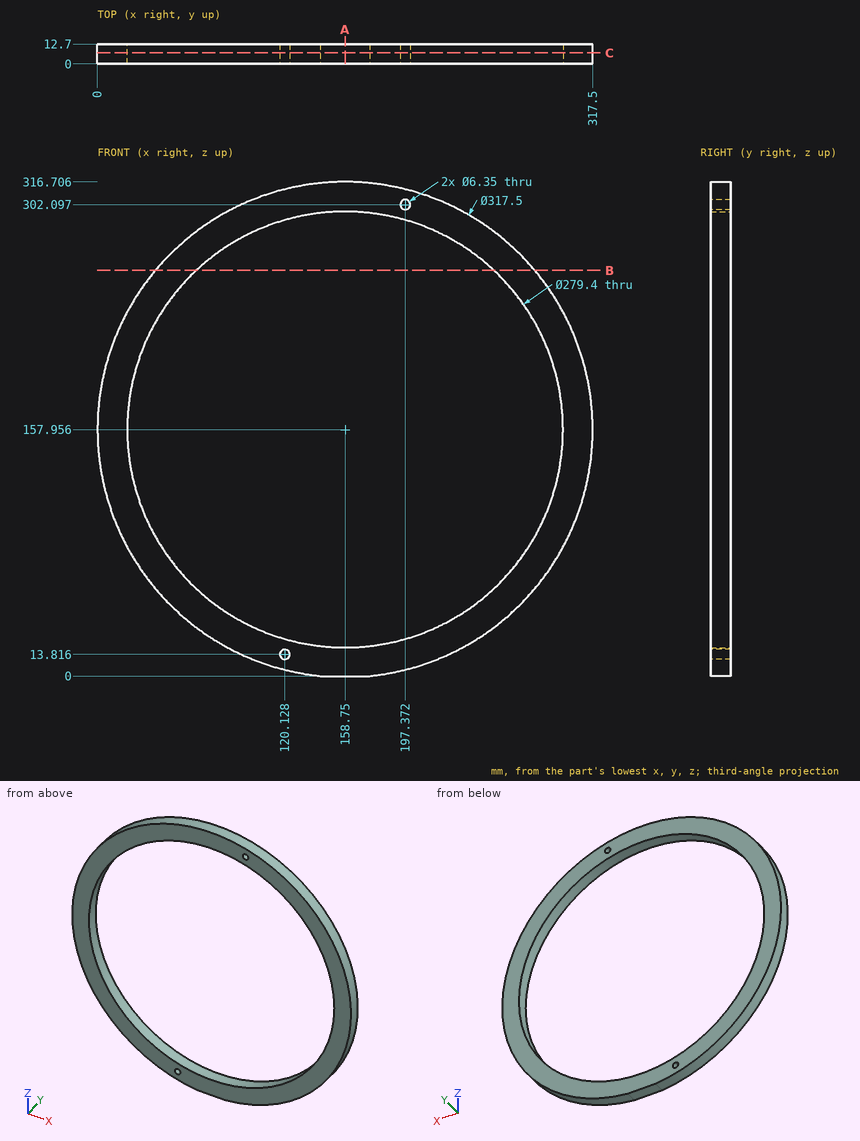
Answer from the drawing. Dimensions are ordinates in mm from the lowest x, y and z of the part. Give positions to 0.01 mm unless a question says otherwise; leave off trailing zeros. Loops run counter-clockwise (first coordinate to the right, second up) from the corner with the lowest first, then second, coordinate; pieces in that order, holes last. Notation, with made-up numbers: (32.25, -32) -> (61.25, -32) arc R29 ccw to (61.25, -10) -> close; hole circle Ø6 at (78, 86). An arc over 180 degrees is marked (long way). Use a Markdown table: item, result.
Q1. Find the intervals of material crossed by line 1 along X through (y, z) = (6.5, 154); line 2 along Z through (x, y) = (88.5, 11) (1 decimal); line 3 along Z through (x, y) = (113, 0.5), in increasing order.
Solved:
| item | result |
|---|---|
| line 1 | x = 0.05 to 19.11, 298.39 to 317.45 |
| line 2 | z = 15.6 to 37.2, 278.7 to 300.3 |
| line 3 | z = 5.94 to 25.96, 289.95 to 309.97 |
Q2. Each of these flat-tipped pins is pushed along its axis until it touches: pin 1 (1 mm diameter, centred on x = 41, y = 1.5, fed in from +Z); pin 2 (6 mm diameter, centred on x = 35.5, y = 11, fed in from -Z) (1 decimal); pin 3 (2 mm diameter, centred on x = 262, y = 8.5, fed in from -Z); pin 4 (5.5 mm diameter, centred on x = 197.37, z = 302.1, fed in from -Y). Where does it stop, or does it pass through?
Solved:
| item | result |
|---|---|
| pin 1 | stops at z = 264.98 |
| pin 2 | stops at z = 54.3 |
| pin 3 | stops at z = 36.52 |
| pin 4 | passes through |
Q3. Section B-B, the plane z = 260 is taken. Determine the outline of the cut face in (x, y).
Solved:
| item | result |
|---|---|
| outline | (37.14, 0) -> (63.34, 0) -> (63.34, 12.7) -> (37.14, 12.7) -> close; (254.16, 0) -> (280.36, 0) -> (280.36, 12.7) -> (254.16, 12.7) -> close |
Q4. Section A-A, the plane x = 158.75 is taken. Determine the outline of the cut face in (y, z).
Solved:
| item | result |
|---|---|
| outline | (0, 0) -> (12.7, 0) -> (12.7, 18.26) -> (0, 18.26) -> close; (0, 297.66) -> (12.7, 297.66) -> (12.7, 316.71) -> (0, 316.71) -> close |
Q5. Section C-C, the plane y = 7 is taken. Count the separate pieces of the cut face and the enclosed holes in it, then the cut area to 3 significant figures.
Solved:
| item | result |
|---|---|
| separate pieces | 1 |
| enclosed holes | 3 |
| area | 17,800 mm^2 |
